```python
from build123d import *

# Parameters (mm, degrees)
REVOLUTION_ANGLE = 85
FILLET_R         = 8
PAD_DEPTH        = 8
POCKET_DEPTH     = 2
CHAMFER_SIZE     = 1
SKETCH005_W      = 3
SKETCH005_H      = 7
POCKET001_DEPTH  = 87.696576
POCKET002_DEPTH  = 78.501
SKETCH007_W      = 3
SKETCH007_H      = 6
POCKET003_DEPTH  = 87.696576


with BuildPart() as part:
    # Sketch → Revolution (revolve, symmetric)
    with BuildSketch(Plane.XY) as revolution_sk:
        with BuildLine():
            ThreePointArc((28, 223.47956), (0, 250), (-28, 223.47956))
            Line((-35.25, 90), (-28, 223.47956))
            Line((-35.25, 90), (-33.25, 90))
            Line((-33.25, 90), (-26.001373, 223.4))
            ThreePointArc((26.001373, 223.4), (0, 248.411154), (-26.001373, 223.4))
            Line((26.001373, 223.4), (33.25, 90))
            Line((33.25, 90), (35.25, 90))
            Line((35.25, 90), (28, 223.47956))
        make_face()
    revolve(axis=Axis((0, 0, 0), (1, 0, 0)), revolution_arc=REVOLUTION_ANGLE / 2)
    revolve(revolution_sk.sketch, axis=Axis((0, 0, 0), (-1, 0, 0)), revolution_arc=REVOLUTION_ANGLE / 2)

    # Fillet
    fillet_edges = [part.edges().sort_by_distance(p)[0] for p in [
        (34.25, 66.35496, 60.803119),
        (-34.25, 66.35496, 60.803119),
    ]]
    fillet(fillet_edges, radius=FILLET_R)

    # Sketch002 (on Face5 of Fillet) → Pad (new body)
    with BuildSketch(Plane(origin=(0, 0, 0), x_dir=(1, 0, 0), z_dir=(0, -0.67559, 0.737277))):
        Polygon((-43.394171, 132.697505), (-46.5, 121.106395), (-33.248819, 107.855214), (-31, 145.091677), align=None)
        Polygon((43.394171, 132.697505), (46.5, 121.106395), (33.248819, 107.855214), (31, 145.091677), align=None)
        Polygon((28, 194.106395), (32, 198.106395), (32, 206.106395), (28, 210.106395), (24, 206.106395), (24, 198.106395), align=None)
        Polygon((-28, 194.106395), (-24, 198.106395), (-24, 206.106395), (-28, 210.106395), (-32, 206.106395), (-32, 198.106395), align=None)
    extrude(amount=-PAD_DEPTH)

    # Sketch003 (on Face47 of Pad) → Pocket (cut)
    with BuildSketch(Plane(origin=(0, 0, 0), x_dir=(1, 0, 0), z_dir=(0, -0.67559, 0.737277))):
        Polygon((35, 146.869795), (45, 97.88), (47.939388, 98.48), (37.939388, 147.469795), align=None)
        Polygon((-47.939388, 98.48), (-45, 97.88), (-35, 146.869795), (-37.939388, 147.469795), align=None)
    extrude(amount=-POCKET_DEPTH, mode=Mode.SUBTRACT)

    # Chamfer
    chamfer_edges = [part.edges().sort_by_distance(p)[0] for p in [
        (42.094426, 93.718526, 85.877207),
        (38.89944, 94.199359, 86.317809),
        (-38.89944, 94.199359, 86.317809),
        (-42.094426, 93.718526, 85.877207),
    ]]
    chamfer(chamfer_edges, length=CHAMFER_SIZE)

    # Sketch005 (on Face6 of Chamfer) → Pocket001 (cut, through all)
    with BuildSketch(Plane(origin=(0, 5.404722, -5.898219), x_dir=(1, 0, 0), z_dir=(0, 0.67559, -0.737277))):
        with Locations((-36.047712, 125.078524)):
            Rectangle(SKETCH005_W, SKETCH005_H)
        with Locations((36.047712, 125.078524)):
            Rectangle(SKETCH005_W, SKETCH005_H)
    extrude(amount=-POCKET001_DEPTH, mode=Mode.SUBTRACT)

    # Sketch006 → Pocket002 (cut, through all)
    with BuildSketch(Plane.YZ.offset(32)):
        Polygon((154.311436, 128.180853), (156.149665, 125.810007), (160.891358, 129.486466), (159.053128, 131.857312), align=None)
    extrude(amount=-POCKET002_DEPTH, mode=Mode.SUBTRACT)

    # Sketch007 (on Face6 of Pocket002) → Pocket003 (cut, through all)
    with BuildSketch(Plane(origin=(0, 5.404722, -5.898219), x_dir=(1, 0, 0), z_dir=(0, 0.67559, -0.737277))):
        with Locations((-35.898523, -126.117473)):
            Rectangle(SKETCH007_W, SKETCH007_H)
        with Locations((35.898523, -126.117473)):
            Rectangle(SKETCH007_W, SKETCH007_H)
    extrude(amount=-POCKET003_DEPTH, mode=Mode.SUBTRACT)


solid = part.part
```
Model file for the job. Use its own axes, mm. Give positions to 0.01 mm unless a question says otherwise; leave off trailing zeros. Write each loop counter-clockwise with the first axis right and the second up, starting at its lowest first coordinate (ties: lowest second). Pieces come first, ordered by that corner, then holes. Notation, with made-up numbers: (89, 30) - (96, 30) arc R25 ccw to (96, 50) - close; hole circle Ø11 at (-19.5, 49). An arc over 180 degrees is marked (long way). One line per question, with ' | ' between items. Start each with the question number.
(1) Wall check: line 1 along X through (y, z) = (182, -85); line 2 along X through (y, z) = (190, 30); line 3 along Z through (x, y) = (14.5, 198.5). Give the ranges that are in metal, low to high. Write a range as from..to.
(2) Slice it at A-A on x = -6.5. Write the cut outline in (y, z).
(3) Pin check, flat tips, straight feed: P1, Ø8, axis at x = 10.5, y = 205, coming from the +Z side; P2, Ø6, axis at y = 162, z = 73, coming from the +X side; P3, Ø1, axis at y = 104, z = 11, coming from the +X side. Stop position of each tip, or through.
(4) Two-plate mould, pull along X, no slides. Class faces 1 (the face through (-30.38, 142.8, 1.48)), 2 (the face through (37.11, 105.13, 90.99)), 3 (the face through (-32.38, 142.84, 1.48)): +X half, -X half, draft (parallel to the pull), parting line (faces both ways), or undercut.
(5) Slice it at B-B on x = 13.5. Write the cut outline in (y, z), plus the area to 3 significant figures.
Results below:
1) line 1: -29.23..-27.23, 27.23..29.23 | line 2: -29.69..-27.69, 27.69..29.69 | line 3: -145.24..-141.89, 141.89..145.24
2) outline: (182.54, -167.27) - (183.76, -168.38) arc R249.24 ccw to (183.76, 168.38) - (182.54, 167.27) arc R247.59 cw to start
3) P1: z = 145.75 | P2: x = 30.65 | P3: x = 34.49
4) face 1: undercut | face 2: +X half | face 3: -X half
5) outline: (180.36, -165.27) - (181.77, -166.56) arc R246.54 ccw to (181.77, 166.56) - (180.36, 165.27) arc R244.64 cw to start | area: 693 mm^2
